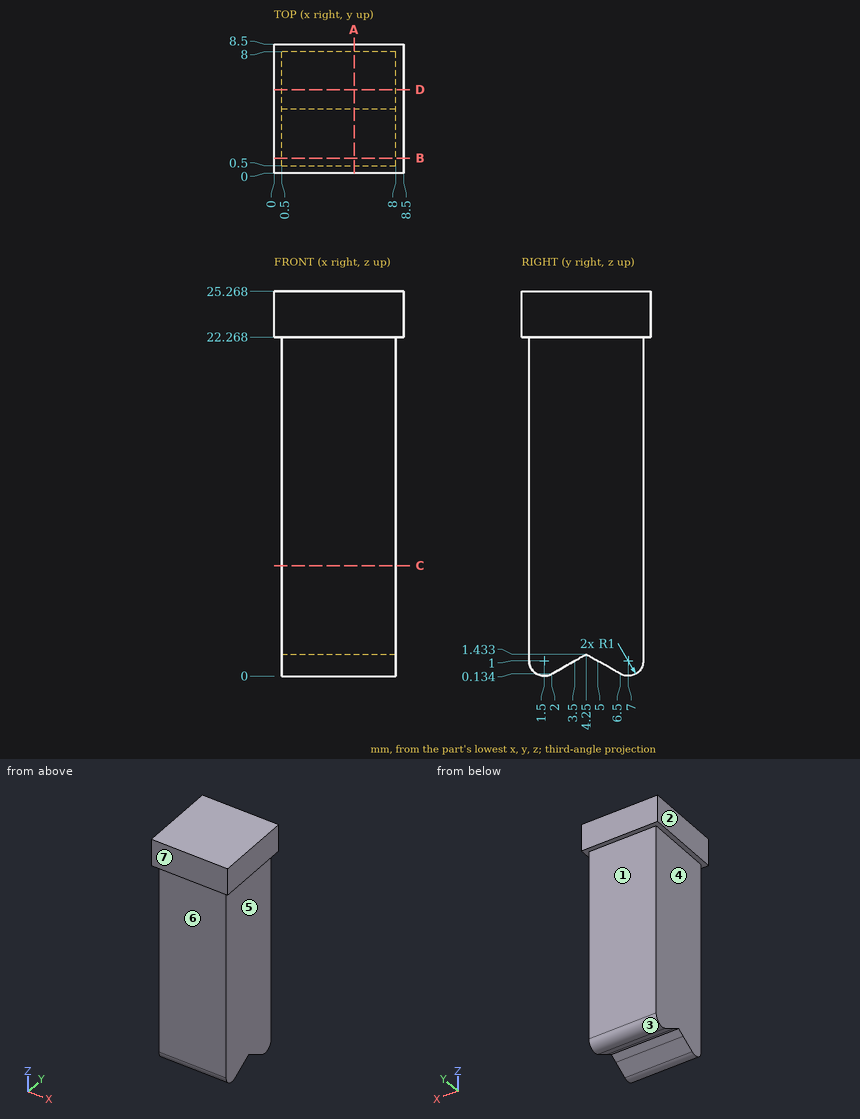
Input: dimensioned drawing with shaded views. Units: mm. Origin: part minimum x, y, z. A direction names the side the tool comes from. Coordinates: 2 decimals unless noted, no trailing zeros. Loops run counter-clockwise (first coordinate to the right, second up) from the corner with the lowest first, then second, coordinate; pieces in that order, holes last. Notation, with made-up numbers: M 4,72.25 L 9,72.25 A11 cw 9,81.25 Z; hole C -30,77.25 d2. An arc over 180 degrees is marked long. Put each result on its own line as item: value.
(1) Cut plane D-D on y = 5.5. Return the cut outline in (x, z), then the cut area to 3 significant figures.
Answer sheet:
outline: M 0,22.27 L 0.5,22.27 L 0.5,0.71 L 8,0.71 L 8,22.27 L 8.5,22.27 L 8.5,25.27 L 0,25.27 Z
area: 187 mm^2
(2) Access query for the marked faces 4, 5, 6 and 7. Directions: +Z, -Z, +X, -X, +Y, -Y. A direction counts if a zero-diameter tool reaches every point of the face in a straight line with its end or side. Return the directions, or none.
Answer sheet:
face 4: -Z, -X, +Y, -Y
face 5: -Z, +X, +Y, -Y
face 6: -Z, +X, -X, -Y
face 7: +Z, -Z, +X, -X, -Y
(3) Material intervals for probe 1 along X at (y, z) = (4.25, 10); probe 2 along Z at (x, y) = (1, 2), sorted ascending.
Answer sheet:
probe 1: x = 0.5 to 8
probe 2: z = 0.13 to 25.27
(4) First-contact query: pin 1 (2 mm diameter, centred on x = 2.5, z = 13, fed in from +Y); pin 2 (3 mm diameter, centred on y = 4, z = 16, fed in from -X); pin 3 (5 mm diameter, centred on y = 5.5, z = 12.5, fed in from +X); pin 4 (4 mm diameter, centred on x = 5.5, y = 6, fed in from -Z). Flat tips, straight axial feed; report the tip coordinate or a pass-through.
Answer sheet:
pin 1: stops at y = 8
pin 2: stops at x = 0.5
pin 3: stops at x = 8
pin 4: stops at z = 0
(5) Draft query along Y for the marked faces 1, 2 and 3. Return one class per face: pulls with the +Y half, pulls with the -Y half, needs draft (parallel to the pull), parting line crosses it, or undercut.
Answer sheet:
face 1: pulls with the +Y half
face 2: needs draft
face 3: undercut
(6) Cut plane B-B on y = 1. Return the cut outline in (x, z), then the cut area to 4 significant figures.
Answer sheet:
outline: M 0,22.27 L 0.5,22.27 L 0.5,0.13 L 8,0.13 L 8,22.27 L 8.5,22.27 L 8.5,25.27 L 0,25.27 Z
area: 191.5 mm^2
(7) Cut plane C-C on z = 7.25. Return the cut outline in (x, y), then the cut area to 4 significant figures.
Answer sheet:
outline: M 0.5,0.5 L 8,0.5 L 8,8 L 0.5,8 Z
area: 56.25 mm^2
(8) Cut plane A-A on x = 5.25. Return the cut outline in (y, z), then the cut area to 3 significant figures.
Answer sheet:
outline: M 0,22.27 L 0.5,22.27 L 0.5,1 A1 ccw 2,0.13 L 4.25,1.43 L 6.5,0.13 A1 ccw 8,1 L 8,22.27 L 8.5,22.27 L 8.5,25.27 L 0,25.27 Z
area: 189 mm^2
